Geometry check sheet. Reference: the model listing, model coordinates, mm. A direction names the side the tool comes from. Round coordinates to 2 decimals unless told otherwise and drop trailing zeros. Write each loop counter-clockwise with the first axis right and the second up, starting at its lowest first coordinate (ties: lowest second). Pieces come first, ordered by that corner, then holes. Notation, with made-up numbers: M 81.5,36.25 L 121.5,36.25 A31 cw 121.5,69.25 Z; hole C -23,25.25 d2. An arc over 180 degrees is marked long. Put each result on its own line as item: value. Start each with the question number.
(1) Section check D-D on y = 56.5. Record the cut outline in (x, z).
(2) Section check A-A on y = 47. Record the cut outline in (x, z).
(3) Mould release check, pull along Y, two halves, no side actions. Record for faces 4 (the flat face through (0, 23, 18)), 5 (the flat face through (39.1, 53.9, 25.6)), 6 (the flat face through (42, 53, 18)): pulls with the +Y half, pulls with the -Y half, needs draft (parallel to the pull), parting line crosses it, or undercut.
(4) Material ranges on probe 1 along Z at (x, y) = (20, 52.5); probe 2 along Z at (x, y) = (33.5, 52.5); probe 3 along Y at (x, z) = (11.5, 9), recorded low to high.
(5) Section check C-C on z = 9. Record the cut outline in (x, y), then the cut area to 3 significant figures.
(6) Tool access check on faces 1 (the cylindrical face through (14.81, 50.893, 9.211)), 2 (the flat face through (24, 53, 18)), 3 (the cylindrical face through (32.46, 51.35, 10.25)). Record the directions out of +Z, -Z, +X, -X, +Y, -Y that give a thin tool (end or side, any length) a straight path to the whole face; none if there is none.
(7) Gauge pin test, flat ends, axial feed: pin 1 (1.9 mm diameter, centred on y = 52.5, z = 9, fed in from -X); pin 2 (16 mm diameter, centred on y = 54, z = 26.5, fed in from -X); pin 3 (4.5 mm diameter, centred on y = 52.5, z = 27, fed in from +X); pin 4 (12 mm diameter, centred on x = 30.5, z = 21, fed in from -Y). Record the tip position at first contact, or that the pin passes through.
(8) Section check B-B on x = 41. Record the cut outline in (y, z), then the cut area to 3 significant figures.
Autodesk Inventor part; units mm, degrees
ref_plane "Arbeitsebene1" through (42.5, 0, 0) normal (1, 0, 0) x (0, 0, -1)
ref_plane "Arbeitsebene3" through (0, 0, 27) normal (0, 0, 1) x (1, 0, 0)
ref_plane "Arbeitsebene4" through (0, 0, 9) normal (0, 0, -1) x (-1, 0, 0)
sketch "Skizze1" plane through (0, 0, 0) normal (0, 0, 1) x (1, 0, 0)
  line L0 (0, 0) -> (50, 0)
  line L1 (50, 0) -> (50, 45)
  line L2 (35, 60) -> (15, 60)
  line L3 (0, 45) -> (0, 0)
  circle A0 centre (25, 28) radius 17.5
  line L4 (25, 28) -> (25, 0) construction
  line L5 (0, 45) -> (15, 60)
  line L6 (35, 60) -> (50, 45)
  line L7 (24, 60) -> (26, 60)
  line L8 (26, 60) -> (26, 28)
  line L9 (26, 28) -> (24, 28)
  line L10 (24, 28) -> (24, 60)
  point P0 (50, 60)
  point P1 (0, 60)
  point P2 (25, 60)
  dimension "d0" = 50
  dimension "d1" = 35
  dimension "d2" = 60
  dimension "d3" = 15
  dimension "d4" = 15
  dimension "d5" = 15
  dimension "d6" = 15
  dimension "d7" = 28
  dimension "d10" = 2
extrude "Extrusion1" add sketch "Skizze1" along normal blind 36 contours L3 L5 L2 L10 A0 L8 L6 L1 L0 | L2 L8 A0 L10
extrude "Extrusion2" cut sketch "Skizze1" along normal up to surface (36 mm away) contours L2 L8 A0 L10 | A0 L8 L9 L10 picked at (24.8888, 33.8323)
ref_plane "Arbeitsebene1" through (42.5, 0, 0) normal (1, 0, 0) x (0, 0, -1)
sketch "Skizze3" plane through (42.5, 0, 0) normal (1, 0, 0) x (0, 0, -1)
  line L0 (0, 60) -> (-36, 60) construction
  line L1 (0, 45) -> (-36, 45) construction
  line L2 (-36, 45) -> (-36, 60) construction
  line L3 (-36, 52.5) -> (0, 52.5) construction
  line L4 (0, 45) -> (0, 60) construction
  point P0 (0, 0)
  point P1 (-18, 52.5)
  point P2 (-27, 52.5)
  point P3 (-9, 52.5)
  dimension "d44" = 9
  dimension "d45" = 9
ref_plane "Arbeitsebene2" through (0, 0, 18) normal (0, 0, 1) x (1, 0, 0)
ref_plane "Arbeitsebene3" through (0, 0, 27) normal (0, 0, 1) x (1, 0, 0)
ref_plane "Arbeitsebene4" through (0, 0, 9) normal (0, 0, -1) x (-1, 0, 0)
sketch "Skizze5" plane through (50, 0, 36) normal (1, 0, 0) x (0, 0, -1)
  line L0 (18, -12) -> (18, 72) construction
  line L1 (9, -12) -> (9, 72) construction
  line L2 (27, 72) -> (27, -12) construction
  point P0 (36, 0)
  dimension "Hole_Dist2Center" = 9
  dimension "d37" = 9
hole "Bohrung2" at (42.5, 52.5, 27) at (42.5, 52.5, 9) direction (-1, 0, 0) diameter 3.4 depth 18.5 counterbore diameter 6.5 counterbore depth 3.4
delete faces "Fläche löschen1" heal yes whole lump no faces at (42.5, 51.6084, 27.6154) (42.5, 51.6084, 9.6154)
sketch "Skizze4" plane through (24, 45.4714, 0) normal (1, 0, 0) x (0, 0, -1)
  line L0 (-18, 7.0286) -> (-27, 7.0286) construction
  line L1 (-27, -57.4714) -> (-27, 26.5286) construction
  line L2 (-9, 26.5286) -> (-9, -57.4714) construction
  point P0 (0, -45.4714)
  point P1 (-9, 7.0286)
hole "Bohrung3" at (24, 52.5, 27) at (24, 52.5, 9) direction (-1, 0, 0) diameter 3.242 end through all
sketch "Skizze7" plane through (0, 0, 0) normal (0, 0, -1) x (-1, 0, 0)
  line L0 (-43.9281, 6.4649) -> (-5.9676, 6.4649) construction
  line L1 (0, 0) -> (-50, 0) construction
  line L2 (-25, 0) -> (-24.9479, 6.4649) construction
  line L3 (0, 45) -> (0, 0) construction
  line L4 (-50, 0) -> (-50, 45) construction
  circle A0 centre (-43.9281, 6.4649) radius 2.5 construction
  circle A1 centre (-5.9676, 6.4649) radius 2.5 construction
  dimension "d50" = 50
  dimension "d51" = 5
equation "\"d0\" = Fixation_Width"
equation "\"d11\" = Fixation_Thickness"
equation "\"Fixation_Thickness\" = 40"
equation "\"Fixation_Width\" = 50"
equation "\"FixationHole_Dist\" = 28"
equation "\"d21\" = -0.5 * d5"
properties part number "MotorFixation_ParallelMecha_Holder"
Answers follow:
1. outline: M 11.5,0 L 24,0 L 24,36 L 11.5,36 Z; M 26,0 L 38.5,0 L 38.5,36 L 26,36 Z
2. outline: M 2,0 L 24,0 L 24,36 L 2,36 Z; M 26,0 L 48,0 L 48,36 L 26,36 Z
3. face 4: needs draft
3. face 5: undercut
3. face 6: pulls with the +Y half
4. probe 1: z = 0 to 7.38, 10.62 to 25.38, 28.62 to 36
4. probe 2: z = 0 to 7.3, 10.7 to 25.3, 28.7 to 36
4. probe 3: y = 0 to 16.86, 39.14 to 50.88, 54.12 to 56.5
5. outline: M 0,0 L 50,0 L 50,45 L 45.75,49.25 L 39.1,49.25 L 39.1,50.8 L 26,50.8 L 26,45.47 A17.5 cw long 24,45.47 L 24,50.88 L 5.88,50.88 L 0,45 Z; M 9.12,54.12 L 24,54.12 L 24,60 L 15,60 Z; M 26,54.2 L 39.1,54.2 L 39.1,55.75 L 39.25,55.75 L 35,60 L 26,60 Z
5. area: 1,660 mm^2
6. face 1: +X, -X
6. face 2: +Z, -Z, +Y
6. face 3: +X
7. pin 1: passes through
7. pin 2: stops at x = 1
7. pin 3: stops at x = 39.1
7. pin 4: stops at y = 0
8. outline: M 0,0 L 20.91,0 L 20.91,36 L 0,36 Z; M 35.09,0 L 54,0 L 54,6.12 A3.25 cw long 54,11.88 L 54,24.12 A3.25 cw long 54,29.88 L 54,36 L 35.09,36 Z
8. area: 1,380 mm^2
